from build123d import *

# Parameters (mm, degrees)
SKETCH1_R                     = 4.5
BOSS_EXTRUDE1_DEPTH           = 11
CUT_EXTRUDE1_START            = -2
CUT_EXTRUDE1_DEPTH            = 2
SKETCH3_R                     = 1.4999999999999996
BOSS_EXTRUDE2_DEPTH           = 1
BOSS_EXTRUDE2_DRAFT           = 10.000000000000021
BOSS_EXTRUDE2_PROFILE_2_DEPTH = 1
BOSS_EXTRUDE2_PROFILE_2_DRAFT = 10.000000000000021
BOSS_EXTRUDE2_PROFILE_3_DEPTH = 1
BOSS_EXTRUDE2_PROFILE_3_DRAFT = 10.000000000000021
SKETCH3_R_2                   = 1.5000000000000002
BOSS_EXTRUDE2_PROFILE_4_DEPTH = 1
BOSS_EXTRUDE2_PROFILE_4_DRAFT = 10.000000000000021
SKETCH4_R                     = 1.5999999999999999
CUT_EXTRUDE2_DEPTH            = 24.7815054191277
CUT_EXTRUDE3_DEPTH            = 24.7815054191277
CUT_EXTRUDE3_DEPTH_BACK       = 5
SKETCH5_R                     = 2.7999999999999994
SKETCH5_R_2                   = 2.8
CUT_EXTRUDE4_DEPTH            = 3
CUT_EXTRUDE5_START            = -2
CUT_EXTRUDE5_DEPTH            = 2
BOSS_EXTRUDE3_DEPTH           = 1
CUT_EXTRUDE6_DEPTH            = 1
FILLET1_R                     = 1
CUT_EXTRUDE7_DEPTH            = 2


with BuildPart() as part:
    # Sketch1 → Boss-Extrude1 (new body)
    with BuildSketch(Plane.XY):
        with BuildLine():
            ThreePointArc((3.993464047921404, -12.371428571428574), (13.000000000000002, 0), (3.9934640479214014, 12.371428571428574))
            ThreePointArc((3.9934640479214014, 12.371428571428574), (2.9081167199998763, 15.346426249302382), (-4.07e-15, 16.6))
            ThreePointArc((-4.07e-15, 16.6), (-2.908116719999883, 15.346426249302382), (-3.9934640479214067, 12.371428571428574))
            ThreePointArc((-3.9934640479214067, 12.371428571428574), (-13.000000000000002, 1.59e-15), (-3.993464047921404, -12.371428571428574))
            ThreePointArc((-3.993464047921404, -12.371428571428574), (-2.90811671999988, -15.346426249302382), (0, -16.6))
            ThreePointArc((0, -16.6), (2.90811671999988, -15.346426249302382), (3.993464047921404, -12.371428571428574))
        make_face()
        Circle(SKETCH1_R, mode=Mode.SUBTRACT)
        with BuildLine():
            ThreePointArc((1.5870475987269075, -12.396825396825397), (4.5e-16, -11), (-1.587047598726907, -12.396825396825397))
            ThreePointArc((-1.587047598726907, -12.396825396825397), (-2.6e-16, -14.2), (1.5870475987269075, -12.396825396825397))
        make_face(mode=Mode.SUBTRACT)
        with BuildLine():
            ThreePointArc((-1.5870475987270802, 12.396825396825376), (-4.89e-15, 10.99999999999983), (1.5870475987267345, 12.396825396825419))
            ThreePointArc((1.5870475987267345, 12.396825396825419), (-2.28e-15, 14.199999999999829), (-1.5870475987270802, 12.396825396825376))
        make_face(mode=Mode.SUBTRACT)
    extrude(amount=BOSS_EXTRUDE1_DEPTH)

    # Sketch2 → Cut-Extrude1 (cut)
    with BuildSketch(Plane.XY.offset(11).offset(CUT_EXTRUDE1_START)):
        with BuildLine():
            Line((-9.998792207106897, -8.30807765966944), (1.5, -4.242640687119285))
            Line((1.5, -4.242640687119285), (1.5, 4.242640687119285))
            Line((1.5, 4.242640687119285), (-9.998792207106897, 8.30807765966944))
            ThreePointArc((-9.998792207106897, 8.30807765966944), (-13.000000000000002, 1.59e-15), (-9.998792207106897, -8.30807765966944))
        make_face()
    extrude(amount=CUT_EXTRUDE1_DEPTH, mode=Mode.SUBTRACT)


with BuildPart() as boss_extrude2_tool:
    # Sketch3 → Boss-Extrude2 (with draft: the straight prism first)
    with BuildSketch(Plane.XY.offset(11)):
        with Locations((-5.5, -9)):
            Circle(SKETCH3_R)
    extrude(amount=BOSS_EXTRUDE2_DEPTH)
    # Boss-Extrude2: the draft: its side faces are tilted about the plane it starts from
    boss_extrude2_sides = [boss_extrude2_tool.faces().sort_by_distance(p)[0] for p in [
        (-7, -9, 11.5),
    ]]
    draft(boss_extrude2_sides, Plane.XY.offset(11), BOSS_EXTRUDE2_DRAFT)


with BuildPart() as part_1:
    add(part.part)

    # Boss-Extrude2: add boss_extrude2_tool
    add(boss_extrude2_tool.part)


with BuildPart() as boss_extrude2_profile_2_tool:
    # Sketch3 → Boss-Extrude2 profile 2 (with draft: the straight prism first)
    with BuildSketch(Plane.XY.offset(11)):
        with Locations((5.5, -9)):
            Circle(SKETCH3_R)
    extrude(amount=BOSS_EXTRUDE2_PROFILE_2_DEPTH)
    # Boss-Extrude2 profile 2: the draft: its side faces are tilted about the plane it starts from
    boss_extrude2_profile_2_sides = [boss_extrude2_profile_2_tool.faces().sort_by_distance(p)[0] for p in [
        (4, -9, 11.5),
    ]]
    draft(boss_extrude2_profile_2_sides, Plane.XY.offset(11), BOSS_EXTRUDE2_PROFILE_2_DRAFT)


with BuildPart() as part_2:
    add(part_1.part)

    # Boss-Extrude2 profile 2: add boss_extrude2_profile_2_tool
    add(boss_extrude2_profile_2_tool.part)


with BuildPart() as boss_extrude2_profile_3_tool:
    # Sketch3 → Boss-Extrude2 profile 3 (with draft: the straight prism first)
    with BuildSketch(Plane.XY.offset(11)):
        with Locations((5.499999999999998, 9)):
            Circle(SKETCH3_R)
    extrude(amount=BOSS_EXTRUDE2_PROFILE_3_DEPTH)
    # Boss-Extrude2 profile 3: the draft: its side faces are tilted about the plane it starts from
    boss_extrude2_profile_3_sides = [boss_extrude2_profile_3_tool.faces().sort_by_distance(p)[0] for p in [
        (4, 9, 11.5),
    ]]
    draft(boss_extrude2_profile_3_sides, Plane.XY.offset(11), BOSS_EXTRUDE2_PROFILE_3_DRAFT)


with BuildPart() as part_3:
    add(part_2.part)

    # Boss-Extrude2 profile 3: add boss_extrude2_profile_3_tool
    add(boss_extrude2_profile_3_tool.part)


with BuildPart() as boss_extrude2_profile_4_tool:
    # Sketch3 → Boss-Extrude2 profile 4 (with draft: the straight prism first)
    with BuildSketch(Plane.XY.offset(11)):
        with Locations((-5.500000000000003, 9)):
            Circle(SKETCH3_R_2)
    extrude(amount=BOSS_EXTRUDE2_PROFILE_4_DEPTH)
    # Boss-Extrude2 profile 4: the draft: its side faces are tilted about the plane it starts from
    boss_extrude2_profile_4_sides = [boss_extrude2_profile_4_tool.faces().sort_by_distance(p)[0] for p in [
        (-7, 9, 11.5),
    ]]
    draft(boss_extrude2_profile_4_sides, Plane.XY.offset(11), BOSS_EXTRUDE2_PROFILE_4_DRAFT)


with BuildPart() as part_4:
    add(part_3.part)

    # Boss-Extrude2 profile 4: add boss_extrude2_profile_4_tool
    add(boss_extrude2_profile_4_tool.part)

    # Sketch4 → Cut-Extrude2 (cut, through all)
    with BuildSketch(Plane.XY.offset(11)):
        with Locations((5.65685424949239, -5.656854249492369)):
            Circle(SKETCH4_R)
        with Locations((-5.65685424949239, 5.656854249492373)):
            Circle(SKETCH4_R)
    extrude(amount=-CUT_EXTRUDE2_DEPTH, mode=Mode.SUBTRACT)

    # Sketch5 → Cut-Extrude3 (cut, two sides: drawn at the far end of the back side and taken through both)
    with BuildSketch(Plane.XY.offset(11).offset(-CUT_EXTRUDE3_DEPTH_BACK)):
        with Locations(Location((5.65685424949239, -5.656854249492369, 0), (0, 0, 240.938574299))):
            Circle(SKETCH5_R)
        with Locations(Location((-5.656854249492392, 5.656854249492367, 0), (0, 0, 138.454024878))):
            Circle(SKETCH5_R_2)
    extrude(amount=CUT_EXTRUDE3_DEPTH + CUT_EXTRUDE3_DEPTH_BACK, mode=Mode.SUBTRACT)

    # Sketch6 → Cut-Extrude4 (cut)
    with BuildSketch(Plane(origin=(0, 0, 0), x_dir=(-1, 0, 0), z_dir=(0, 0, -1))):
        Polygon((9.73e-15, 9.366838492538095), (2.800000000000004, 10.983419246269044), (2.800000000000004, 14.216580753730957), (1.041e-14, 15.833161507461904), (-2.7999999999999936, 14.21658075373095), (-2.7999999999999936, 10.98341924626905), align=None)
        Polygon((8.7e-16, -9.366838492538093), (-2.7999999999999994, -10.983419246269044), (-2.7999999999999994, -14.216580753730952), (-7.6e-16, -15.833161507461904), (2.7999999999999994, -14.216580753730952), (2.8000000000000003, -10.983419246269046), align=None)
    extrude(amount=-CUT_EXTRUDE4_DEPTH, mode=Mode.SUBTRACT)

    # Sketch7 → Cut-Extrude5 (cut)
    with BuildSketch(Plane.XY.offset(9).offset(CUT_EXTRUDE5_START)):
        with BuildLine():
            Line((-4.5, 5.5e-16), (-13.000000000000004, 1.59e-15))
            ThreePointArc((-13.000000000000004, 1.59e-15), (-12.226698219314768, -4.4167692552141835), (-9.998792207106897, -8.30807765966944))
            Line((-9.998792207106897, -8.30807765966944), (1.4999999999999987, -4.242640687119285))
            ThreePointArc((1.4999999999999987, -4.242640687119285), (-2.598076211353315, -3.6742346141747677), (-4.5, 5.5e-16))
        make_face()
    extrude(amount=CUT_EXTRUDE5_DEPTH, mode=Mode.SUBTRACT)

    # Sketch8 → Boss-Extrude3 (add)
    with BuildSketch(Plane.XY.offset(11)):
        with BuildLine():
            Line((8.000000000000002, 10.2469507659596), (8.000000000000002, -4.123991570751015))
            ThreePointArc((8.000000000000002, -4.123991570751015), (8.456854249492391, -5.656854249492369), (8.000000000000002, -7.189716928233723))
            Line((8.000000000000002, -7.189716928233723), (8.000000000000002, -10.2469507659596))
            ThreePointArc((8.000000000000002, -10.2469507659596), (13.000000000000002, 0), (8.000000000000002, 10.2469507659596))
        make_face()
    extrude(amount=BOSS_EXTRUDE3_DEPTH)

    # Sketch9 → Cut-Extrude6 (cut)
    with BuildSketch(Plane(origin=(0, 0, 0), x_dir=(-1, 0, 0), z_dir=(0, 0, -1))):
        with BuildLine():
            Line((5.740316883347941, -7.154530445721011), (8.45804460872515, -9.87225817109821))
            ThreePointArc((8.45804460872515, -9.87225817109821), (9.192388155425135, -9.192388155425098), (9.872258171098244, -8.458044608725112))
            Line((9.872258171098244, -8.458044608725112), (7.154530445721033, -5.740316883347915))
            ThreePointArc((7.154530445721033, -5.740316883347915), (4.596194077712568, -4.59619407771255), (5.740316883347941, -7.154530445721011))
        make_face()
    extrude(amount=-CUT_EXTRUDE6_DEPTH, mode=Mode.SUBTRACT)

    # Fillet1
    fillet1_edges = [part_4.edges().sort_by_distance(p)[0] for p in [
        (-3.993464047921405, -12.371428571428574, 5.5),
        (-3.9934640479214067, 12.371428571428574, 5.5),
        (3.9934640479214023, 12.371428571428574, 5.5),
        (3.9934640479214036, -12.371428571428574, 5.5),
        (-4.5, 7.8e-16, 8),
        (-13.000000000000005, 1.59e-15, 8),
        (8.000000000000002, -10.2469507659596, 11.5),
        (8.000000000000002, 10.2469507659596, 11.5),
        (-5.7403168833479405, -7.1545304457210115, 0.5),
        (-7.154530445721033, -5.740316883347915, 0.5),
        (-9.998792207106899, -8.30807765966944, 9),
        (-9.998792207106895, 8.30807765966944, 10),
    ]]
    fillet(fillet1_edges, radius=FILLET1_R)

    # Sketch10 → Cut-Extrude7 (cut)
    with BuildSketch(Plane(origin=(0, 0, 0), x_dir=(-1, 0, 0), z_dir=(0, 0, -1))):
        with BuildLine():
            Line((5.500000000000001, 3.7527767497325657), (7.058845726811989, 2.8527767497325622))
            ThreePointArc((7.058845726811989, 2.8527767497325622), (7.424871130596426, 1.4867513459481236), (6.058845726811987, 1.120725942163687))
            Line((6.058845726811987, 1.120725942163687), (4.499999999999998, 2.0207259421636885))
            ThreePointArc((4.499999999999998, 2.0207259421636885), (4.13397459621556, 3.3867513459481287), (5.500000000000001, 3.7527767497325657))
        make_face()
    extrude(amount=-CUT_EXTRUDE7_DEPTH, mode=Mode.SUBTRACT)


solid = part_4.part
Work out the finished part from the listing and answer in its coordinate system (mm). A direction names the side the tool comes from. Coordinates: 2 decimals unless noted, no trailing zeros. Loops run counter-clockwise (first coordinate to the right, second up) from the corner with the lowest first, then second, coordinate; pieces in that order, holes last. Notation, with made-up numbers: M 1.5,36.25 L 53.5,36.25 A19 ccw 53.5,58.25 Z; hole C 87,24 d1. An arc over 180 degrees is marked long. Answer in a Markdown table with one row per item. Add a question column.
1. A tool of negligible diameter and unlimited length cuts with its end or side. For faces 4 (the cylindrical face through (0, -14.2, 6.9)), 5 (the flat face through (1.42, -15.014, 1.479)), 6 (the flat face through (-0.649, 5.003, 9.986)), from which of +Z, -Z, +X, -X, +Y, -Y can it reach the whole face along a straight path? Write none if from no direction.
2. The mould has two halves that part along Y. Classify faces 1 (the cylindrical face through (-4.976, 8.373, 8.291)), 2 (the flat face through (8, 2, 11.5)), 3 (the cylindrical face through (0.1, 16.6, 5.4)): pulls with the +Y half, pulls with the -Y half, needs draft (parallel to the pull), parting line crosses it, or undercut.
3. Find section A-A, the plane x = 5.5. Write down the section's boundary in (y, z).
4. Consider L1, parallel to Y at x = 0.5, z = 2; L2, parallel to Y at x = 0, z = 8.75; L3, parallel to Z at x = -1, y = -5.5. Determine where each line is inside the solid, lowest interval first.
5. Flat-ended cylindrical pins translate along their axes: P1, Ø4, axis at y = -7, z = 1.5, coming from the -X side; P2, Ø3, axis at x = -8.5, y = 5, coming from the +Z side; P3, Ø3, axis at x = -2, y = 7, coming from the +Z side. Find the tip coordinate at first contact, or state that the pin passes through.
6. Find section B-B, the plane y = -3.5. Write down the section's boundary in (x, z).
7. Find section C-C, the plane z = 6.5. State how many separate pieces and enclosed holes the cut face has, then the cut area to 3 significant figures.
Reported:
| question | item | result |
|---|---|---|
| 1 | face 4 | +Z, -Z |
| 1 | face 5 | -Z |
| 1 | face 6 | +Z, -X |
| 2 | face 1 | undercut |
| 2 | face 2 | needs draft |
| 2 | face 3 | pulls with the +Y half |
| 3 | outline | M -11.78,0 L -7.25,0 L -7.25,6 L -8.45,6 L -8.45,12 L -10.32,12 L -10.5,11 L -11.78,11 Z; M -4.06,0 L 11.78,0 L 11.78,11 L 10.5,11 L 10.32,12 L 7.68,12 L 7.5,11 L -2.86,11 L -2.86,6 L -4.06,6 Z |
| 4 | L1 | y = -16.57 to -15.54, -9.66 to -4.47, 4.47 to 9.66, 15.54 to 16.57 |
| 4 | L2 | y = -16.6 to -14.2, -11 to -4.77, 4.5 to 11, 14.2 to 16.6 |
| 4 | L3 | z = 0 to 11 |
| 5 | P1 | stops at x = -12 |
| 5 | P2 | stops at z = 9 |
| 5 | P3 | stops at z = 11 |
| 6 | outline | M -12.52,0 L -2.83,0 L -2.83,7 L -12.52,7 Z; M 2.83,0 L 12.52,0 L 12.52,12 L 8,12 L 8,11 L 7.44,11 L 7.44,6 L 3.87,6 L 3.87,11 L 2.83,11 Z |
| 7 | separate pieces | 1 |
| 7 | enclosed holes | 5 |
| 7 | area | 449 mm^2 |
